from build123d import *

# Parameters (mm, degrees)
F0_W     = 10
F0_H     = 40
F1_DEPTH = 3
F3_D     = 6
F4_D     = 4


with BuildPart() as f1:
    # F0 (on Top) → F1 (new body)
    with BuildSketch(Plane.XY):
        with Locations((-5, 20)):
            Rectangle(F0_W, F0_H)
    extrude(amount=F1_DEPTH)

    # F3 (through all)
    with Locations(Plane.XY.offset(3)):
        with Locations((-5, 5)):
            Hole(F3_D / 2)

    # F4 (through all)
    with Locations(Plane.XY.offset(3)):
        with Locations((-5, 35)):
            Hole(F4_D / 2)


solid = f1.part
Design review of the part built by this model. Coordinates are the model's own, in mm. Give positions to 0.01 mm unless a question says otherwise; leave off trailing zeros. Loops run counter-clockwise (first coordinate to the right, second up) from the corner with the lowest first, then second, coordinate; pieces in that order, holes last. Notation, with made-up numbers: M 76,74 L 90,74 A34 ccw 90,105 Z; hole C 71.25,29 d9. An arc over 180 degrees is marked long. One line per question, with ' | ' between items. Start each with the question number.
1. To check wall thickness, follow L1, parallel to Y at x = -5, z = 0.85; L2, parallel to Y at x = -2.25, z = 1.75; L3, parallel to Y at x = -4.5, z = 2.55. State the ranges of each line that lie inside material, in increasing order.
2. Add section C-C (z = 1.75). Write out the cut boundary in (x, y), plus the area to 3 significant figures.
3. Add section A-A (y = 5). Write out the cut boundary in (x, z).
4. The part is to be moulded in two halves that separate along X. For faces 1 (the face through (-5, 20, 0)), 2 (the face through (0, 20, 1)), 3 (the face through (-5, 33, 1)), 4 (the face through (-4.35, 2.07, 1.48)), say which applies: released by +X, released by -X, zero draft, split by the parting line, or undercut.
5. Add section D-D (x = -7.5). Write out the cut boundary in (y, z), plus the area to 3 significant figures.
6. Add section B-B (x = -5). Write out the cut boundary in (y, z).
Worked out:
1) L1: y = 0 to 2, 8 to 33, 37 to 40 | L2: y = 0 to 3.8, 6.2 to 40 | L3: y = 0 to 2.04, 7.96 to 33.06, 36.94 to 40
2) outline: M -10,0 L 0,0 L 0,40 L -10,40 Z; hole C -5,5 d6; hole C -5,35 d4 | area: 359 mm²
3) outline: M -10,0 L -8,0 L -8,3 L -10,3 Z; M -2,0 L 0,0 L 0,3 L -2,3 Z
4) face 1: zero draft | face 2: released by +X | face 3: undercut | face 4: undercut
5) outline: M 0,0 L 3.34,0 L 3.34,3 L 0,3 Z; M 6.66,0 L 40,0 L 40,3 L 6.66,3 Z | area: 110 mm²
6) outline: M 0,0 L 2,0 L 2,3 L 0,3 Z; M 8,0 L 33,0 L 33,3 L 8,3 Z; M 37,0 L 40,0 L 40,3 L 37,3 Z
